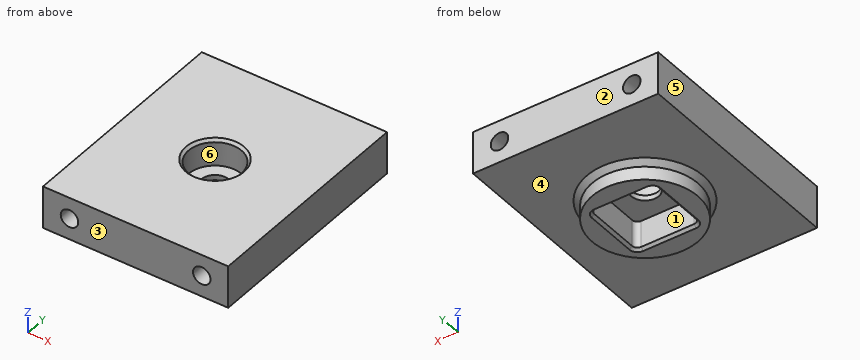
```python
from build123d import *

# Parameters (mm, degrees)
SKETCH_1_W          = 35
SKETCH_1_H          = 42
EXTRUDE_1_DEPTH     = 4
SKETCH_4_R          = 10
EXTRUDE_2_DEPTH     = 3.5
CUT_EXTRUDE_2_DEPTH = 2
SKETCH_6_R          = 2.6
CUT_EXTRUDE_3_DEPTH = 12.5
SKETCH_7_R          = 5
CUT_EXTRUDE_4_DEPTH = 5
CHAMFER_1_SIZE      = 0.5
CHAMFER_2_SIZE      = 0.5
CHAMFER_3_SIZE      = 1
HOLE_WIZARD_M4_1_D  = 3.3


with BuildPart() as part:
    # 草图1 → 凸台-拉伸1 (new body, symmetric)
    with BuildSketch(Plane.XY):
        Rectangle(SKETCH_1_W, SKETCH_1_H)
    extrude(amount=EXTRUDE_1_DEPTH, both=True)

    # 草图4 → 凸台-拉伸2 (add)
    with BuildSketch(Plane(origin=(0, 0, -4), x_dir=(-1, 0, 0), z_dir=(0, 0, -1))):
        Circle(SKETCH_4_R)
        with BuildLine():
            Line((-5, 6), (5, 6))
            ThreePointArc((5, 6), (5.707106781, 5.707106781), (6, 5))
            Line((6, 5), (6, -5))
            ThreePointArc((6, -5), (5.707106781, -5.707106781), (5, -6))
            Line((5, -6), (-5, -6))
            ThreePointArc((-5, -6), (-5.707106781, -5.707106781), (-6, -5))
            Line((-6, -5), (-6, 5))
            ThreePointArc((-6, 5), (-5.707106781, 5.707106781), (-5, 6))
        make_face(mode=Mode.SUBTRACT)
    extrude(amount=EXTRUDE_2_DEPTH)

    # 草图5 → 切除-拉伸2 (cut)
    with BuildSketch(Plane(origin=(0, 0, -4), x_dir=(-1, 0, 0), z_dir=(0, 0, -1))):
        with BuildLine():
            Line((6, -5), (6, 5))
            ThreePointArc((6, 5), (5.707106781, 5.707106781), (5, 6))
            Line((5, 6), (-5, 6))
            ThreePointArc((-5, 6), (-5.707106781, 5.707106781), (-6, 5))
            Line((-6, 5), (-6, -5))
            ThreePointArc((-6, -5), (-5.707106781, -5.707106781), (-5, -6))
            Line((-5, -6), (5, -6))
            ThreePointArc((5, -6), (5.707106781, -5.707106781), (6, -5))
        make_face()
    extrude(amount=-CUT_EXTRUDE_2_DEPTH, mode=Mode.SUBTRACT)

    # 草图6 → 切除-拉伸3 (cut, through all)
    with BuildSketch(Plane.XY.offset(4)):
        Circle(SKETCH_6_R)
    extrude(amount=-CUT_EXTRUDE_3_DEPTH, mode=Mode.SUBTRACT)

    # 草图7 → 切除-拉伸4 (cut)
    with BuildSketch(Plane.XY.offset(4)):
        Circle(SKETCH_7_R)
    extrude(amount=-CUT_EXTRUDE_4_DEPTH, mode=Mode.SUBTRACT)

    # 倒角1
    chamfer_1_edges = [part.edges().sort_by_distance(p)[0] for p in [
        (-5.707106781, 5.707106781, -7.5),
        (0, 6, -7.5),
        (5.707106781, 5.707106781, -7.5),
        (6, 0, -7.5),
        (5.707106781, -5.707106781, -7.5),
        (0, -6, -7.5),
        (-5.707106781, -5.707106781, -7.5),
        (-6, 0, -7.5),
    ]]
    chamfer(chamfer_1_edges, length=CHAMFER_1_SIZE)

    # 倒角2
    chamfer_2_edges = [part.edges().sort_by_distance(p)[0] for p in [
        (-5, 0, 4),
    ]]
    chamfer(chamfer_2_edges, length=CHAMFER_2_SIZE)

    # 倒角3
    chamfer_3_edges = [part.edges().sort_by_distance(p)[0] for p in [
        (10, 0, -4),
    ]]
    chamfer(chamfer_3_edges, length=CHAMFER_3_SIZE)

    # M4 螺纹孔1 (through all)
    with Locations(Plane(origin=(0, 21, 0), x_dir=(1, 0, 0), z_dir=(0, 1, 0))):
        with Locations((-12.5, 0), (12.5, 0)):
            Hole(HOLE_WIZARD_M4_1_D / 2)


solid = part.part
```
Geometry: final body of the model. Coordinates: model frame, mm. Face numbers are marked on the shaded views. A direction names the side the tool comes from. Coordinates: 2 decimals unless noted, no trailing zeros. Loops run counter-clockwise (first coordinate to the right, second up) from the corner with the lowest first, then second, coordinate; pieces in that order, holes last. Notation, with made-up numbers: (-32.5, 10.5) -> (-27.5, 10.5) arc R7 cw to (-27.5, 21.5) -> close; hole circle Ø3 at (50.25, -22.75). An arc over 180 degrees is marked (long way). Use a Markdown table: item, result. Add a question column.
(1) Mould query, pull axis Y, two halves, no side actions, for the marked faces 1, 2 and 3. Classes: pulls with the +Y half, pulls with the -Y half, needs draft (parallel to the pull), parting line crosses it, or undercut.
(2) Section query B-B, the plane y = 0. Return loops of the section in (x, z).
(3) Line query: line 1 along Y through (x, z) = (0, 2.5); line 2 along Y through (x, z) = (0, -1.8); line 3 along Z through (x, y) = (12.5, 0.5). Output: solid intervals per line, ascending.
(4) Pin query (flat end, axial travel): pin 1 Ø8.5 at (x, y) = (0, 0) entering from +Z; pin 2 Ø1.5 at (x, y) = (-7, 9) entering from -Z; pin 3 Ø3 at (x, y) = (9.5, 13) entering from -Z. Return the tip coordinate at first contact, or that it passes through.
(5) Access query for the marked faces 4, 5 and 6. Directions: +Z, -Z, +X, -X, +Y, -Y. A direction counts if a zero-diameter tool reaches every point of the face in a straight line with its end or side. Return the directions, or none.
(6) Section query C-C, the plane x = 12.5. Return loops of the section in (y, z), plus the area to 3 significant figures.
(7) Section query A-A, the plane z = 0. Return loops of the section in (x, y).
(8) Section query D-D, the plane z = -5.5. Return loops of the section in (x, y).
Answer:
| question | item | result |
|---|---|---|
| 1 | face 1 | undercut |
| 1 | face 2 | pulls with the +Y half |
| 1 | face 3 | pulls with the -Y half |
| 2 | outline | (-17.5, -4) -> (-11, -4) -> (-10, -5) -> (-10, -7.5) -> (-6.5, -7.5) -> (-6, -7) -> (-6, -2) -> (-2.6, -2) -> (-2.6, -1) -> (-5, -1) -> (-5, 3.5) -> (-5.5, 4) -> (-17.5, 4) -> close; (2.6, -2) -> (6, -2) -> (6, -7) -> (6.5, -7.5) -> (10, -7.5) -> (10, -5) -> (11, -4) -> (17.5, -4) -> (17.5, 4) -> (5.5, 4) -> (5, 3.5) -> (5, -1) -> (2.6, -1) -> close; hole circle Ø3.3 at (-12.5, 0); hole circle Ø3.3 at (12.5, 0) |
| 3 | line 1 | y = -21 to -5, 5 to 21 |
| 3 | line 2 | y = -21 to -2.6, 2.6 to 21 |
| 3 | line 3 | z = -4 to -1.65, 1.65 to 4 |
| 4 | pin 1 | stops at z = -1 |
| 4 | pin 2 | stops at z = -4.35 |
| 4 | pin 3 | stops at z = -4 |
| 5 | face 4 | -Z |
| 5 | face 5 | +Z, -Z, -X, +Y, -Y |
| 5 | face 6 | +Z |
| 6 | outline | (-21, -4) -> (21, -4) -> (21, -1.65) -> (-21, -1.65) -> close; (-21, 1.65) -> (21, 1.65) -> (21, 4) -> (-21, 4) -> close |
| 6 | area | 197 mm^2 |
| 7 | outline | (-17.5, -21) -> (-14.15, -21) -> (-14.15, 21) -> (-17.5, 21) -> close; (-10.85, -21) -> (10.85, -21) -> (10.85, 21) -> (-10.85, 21) -> close; (14.15, -21) -> (17.5, -21) -> (17.5, 21) -> (14.15, 21) -> close; hole circle Ø10 at (0, 0) |
| 8 | outline | circle Ø20 at (0, 0); hole (-6, -5) arc R1 ccw to (-5, -6) -> (5, -6) arc R1 ccw to (6, -5) -> (6, 5) arc R1 ccw to (5, 6) -> (-5, 6) arc R1 ccw to (-6, 5) -> close |
